Source: CAD feature listing. Evaluate the final solid. Frame: model axes, mm. Give positions to 0.01 mm unless a question says otherwise; leave off trailing zeros. Write each loop counter-clockwise with the first axis right and the second up, starting at its lowest first coordinate (ties: lowest second). Pieces come first, ordered by that corner, then holes. Notation, with made-up numbers: (42, 4.5) - (56, 4.5) arc R21 cw to (56, 25.5) - close; hole circle Ø2 at (-24.75, 70). An arc over 180 degrees is marked (long way). One line per question, with ' | ' between items. Start each with the question number.
(1) Section A-A, the plane x = -36.5. Return loops of the section in (y, z), plus the area to 3 significant figures.
(2) Ray query, line 1 (Z direction, x = -10.5, y = 1.5); line 2 (Z direction, x = 4, y = 1.85); line 3 (Z direction, x = 71, y = 0.5). Return the intervals inside material, ascending. Write a range as [from, to].
(3) Pin query (flat end, axial travel): pin 1 (4 mm diameter, centred on x = 14.5, z = 49.5, fed in from -Y). Return the tip coordinate at first contact, or that it passes through.
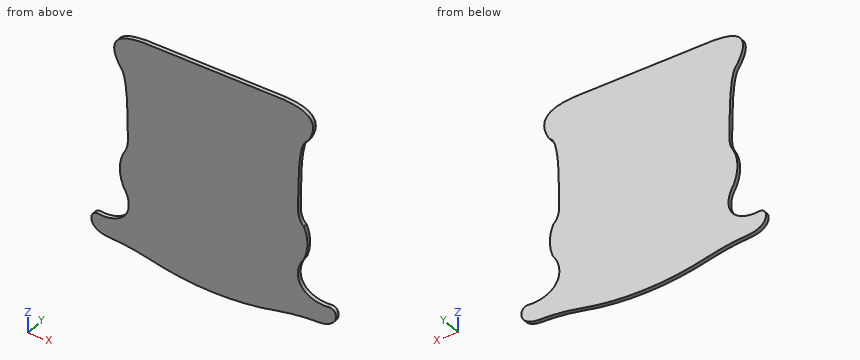
```python
from build123d import *

# Parameters (mm, degrees)
EXTRUDE_1_DEPTH = 3


with BuildPart() as part:
    # 草图1 → 凸台-拉伸1 (new body)
    with BuildSketch(Plane(origin=(0, 0, 0), x_dir=(1, 0, 0), z_dir=(0, 1, 0))):
        with BuildLine():
            Line((0, -85.237738925), (52.08455714, -85.237738925))
            add(Edge.make_bspline(
                [(52.08455714, -85.237738925), (83.131353316, -83.963442969), (70.531928888, -61.056271567)],
                knots=[0, 0, 0, 0.91576418, 0.91576418, 0.91576418], degree=2))
            add(Edge.make_bspline(
                [(64.686979765, -47.335345252), (64.821728452, -48.22885898), (65.093128633, -50.015668979), (65.515155467, -52.234660938), (65.946662506, -53.991070652), (66.337115564, -55.291267739), (66.823261096, -56.557684193), (67.433421369, -57.768689415), (68.186549634, -58.894674775), (69.089475072, -59.904951843), (69.899928779, -60.600614164), (70.397522986, -60.962598407), (70.531928888, -61.056271567)],
                knots=[0, 0, 0, 0, 0.03125, 0.0625, 0.078125, 0.09375, 0.109375, 0.125, 0.140625, 0.15625, 0.171875, 0.177544855, 0.177544855, 0.177544855, 0.177544855], degree=3))
            add(Edge.make_bspline(
                [(67.281190845, 5.878024568), (66.896150113, 5.604067681), (66.17820277, 4.954075775), (65.443341839, 3.984844748), (64.938700468, 3.142617887), (64.602832741, 2.486533462), (64.306406192, 1.811794699), (64.046527331, 1.122513569), (63.82116748, 0.421125393), (63.628358492, -0.290103239), (63.466128453, -1.008847892), (63.332437978, -1.733031566), (63.224920724, -2.461279505), (63.112896984, -3.436590381), (63.04248237, -4.416759867), (63.002674943, -5.39935773), (62.985358555, -6.136929173), (62.977857057, -6.874572053), (62.977765693, -7.612059791), (62.982878051, -8.349301424), (62.991452287, -9.086301707), (63.002218337, -9.823125162), (63.018489212, -10.805396372), (63.040788209, -12.033099303), (63.117509988, -15.961444796), (63.209965223, -19.888985412), (63.30476302, -23.816659201), (63.346660287, -25.535031616), (63.38326061, -27.007933212), (63.421035997, -28.480829039), (63.466381834, -30.199198036), (63.537017062, -32.653910516), (63.649386664, -35.598757346), (63.806392131, -38.54169042), (64.021636354, -41.480498428), (64.260256253, -43.924290625), (64.493829102, -45.874662228), (64.622628022, -46.848447014), (64.686979765, -47.335345252)],
                knots=[0.42243117, 0.42243117, 0.42243117, 0.42243117, 0.4375, 0.453125, 0.4609375, 0.46875, 0.4765625, 0.484375, 0.4921875, 0.5, 0.5078125, 0.515625, 0.5234375, 0.53125, 0.546875, 0.5546875, 0.5625, 0.5703125, 0.578125, 0.5859375, 0.59375, 0.6015625, 0.609375, 0.625, 0.640625, 0.734375, 0.75, 0.765625, 0.7890625, 0.796875, 0.8125, 0.84375, 0.875, 0.90625, 0.9375, 0.96875, 0.984375, 1, 1, 1, 1], degree=3))
            add(Edge.make_bspline(
                [(67.78565705, 30.270686681), (72.435451847, 17.336518953), (67.281190845, 5.878024568)],
                knots=[0.041125556, 0.041125556, 0.041125556, 0.901853171, 0.901853171, 0.901853171], degree=2))
            add(Edge.make_bspline(
                [(67.78565705, 30.270686681), (61.777966314, 38.050300603), (60.870236454, 48.571265725), (67.294682301, 54.787889309)],
                knots=[0.782114211, 0.782114211, 0.782114211, 0.782114211, 1, 1, 1, 1], degree=3))
            add(Edge.make_bspline(
                [(67.294682301, 54.787889309), (70.741983298, 58.123674712), (77.208516837, 60.562602986), (83.906576895, 60.259476119), (84.838000271, 60.163270829)],
                knots=[0, 0, 0, 0, 0.116915593, 0.136015961, 0.136015961, 0.136015961, 0.136015961], degree=3))
            add(Edge.make_bspline(
                [(84.838000271, 60.163270829), (85.146981152, 60.131356669), (85.454953169, 60.093539936), (85.761414982, 60.04983651)],
                knots=[0.136015961, 0.136015961, 0.136015961, 0.136015961, 0.142352122, 0.142352122, 0.142352122, 0.142352122], degree=3))
            add(Edge.make_bspline(
                [(78.685847617, 74.813097523), (82.796268879, 74.469500522), (85.960946813, 73.439665414), (92.408972751, 67.859232167), (92.136253049, 59.602987515), (85.761414982, 60.04983651)],
                knots=[0.020704184, 0.020704184, 0.020704184, 0.020704184, 0.398408746, 0.457074244, 0.967673839, 0.967673839, 0.967673839, 0.967673839], degree=3))
            ThreePointArc((78.685847617, 74.813097523), (62.72522618, 76.083545277), (46.990944234, 79.047975372))
            ThreePointArc((46.990944234, 79.047975372), (23.665112301, 83.299995302), (0, 84.761695887))
            Line((0, 84.761695887), (0, -85.237738925))
        make_face()
        with BuildLine():
            Line((-52.08455714, -85.237738925), (0, -85.237738925))
            Line((0, -85.237738925), (0, 84.761695887))
            ThreePointArc((0, 84.761695887), (-24.143998295, 83.356825814), (-47.941899914, 79.047975372))
            ThreePointArc((-47.941899914, 79.047975372), (-62.863562899, 76.194384461), (-77.997336876, 74.864763259))
            add(Edge.make_bspline(
                [(-77.997336876, 74.864763259), (-82.495528452, 74.563753901), (-85.819969627, 73.561673882), (-92.303254227, 67.950726086), (-92.148043047, 60.049699914), (-86.326016832, 60.03052313)],
                knots=[0, 0, 0, 0, 0.398408746, 0.457074244, 0.95214781, 0.95214781, 0.95214781, 0.95214781], degree=3))
            add(Edge.make_bspline(
                [(-84.476216485, 60.232119747), (-85.0964702, 60.188510883), (-85.714404489, 60.121269756), (-86.326016832, 60.03052313)],
                knots=[0.130603984, 0.130603984, 0.130603984, 0.130603984, 0.143267662, 0.143267662, 0.143267662, 0.143267662], degree=3))
            add(Edge.make_bspline(
                [(-67.726534157, 54.787889309), (-71.173835153, 58.123674712), (-77.383070006, 60.465559796), (-83.805773382, 60.279257331), (-84.476216485, 60.232119747)],
                knots=[0, 0, 0, 0, 0.116915593, 0.130603984, 0.130603984, 0.130603984, 0.130603984], degree=3))
            add(Edge.make_bspline(
                [(-67.318940817, 31.510044314), (-62.135044836, 39.136673255), (-61.6373547, 48.895686695), (-67.726534157, 54.787889309)],
                knots=[0.793484807, 0.793484807, 0.793484807, 0.793484807, 1, 1, 1, 1], degree=3))
            add(Edge.make_bspline(
                [(-67.318940817, 31.510044314), (-73.265342886, 16.40111188), (-65.978257792, 3.284039205)],
                knots=[0, 0, 0, 1, 1, 1], degree=2))
            add(Edge.make_bspline(
                [(-65.637935545, -47.335345136), (-65.373308793, -45.388720399), (-64.924382386, -41.484539572), (-64.643005293, -36.57962883), (-64.490248654, -32.653889947), (-64.374999228, -28.726358209), (-64.257498755, -23.816569768), (-64.116872777, -17.924883735), (-64.009829941, -13.015026184), (-63.947711012, -9.577682419), (-63.927494686, -7.612641533), (-63.933645618, -5.646217447), (-64.01771328, -3.681321264), (-64.270091341, -1.731417529), (-64.514844339, -0.526384591), (-64.771670226, 0.42231228), (-64.996859302, 1.123821794), (-65.256715294, 1.813004408), (-65.553427674, 2.487173233), (-65.802759649, 2.973687329), (-65.950639045, 3.235914899), (-65.978257792, 3.284039205)],
                knots=[0, 0, 0, 0, 0.0625, 0.125, 0.15625, 0.1875, 0.25, 0.3125, 0.375, 0.40625, 0.421875, 0.4375, 0.46875, 0.484375, 0.5, 0.5078125, 0.515625, 0.5234375, 0.53125, 0.5390625, 0.540827672, 0.540827672, 0.540827672, 0.540827672], degree=3))
            add(Edge.make_bspline(
                [(-67.844738769, -56.659038975), (-67.828076267, -56.622229396), (-67.719460833, -56.379300174), (-67.532147702, -55.924331546), (-67.301765295, -55.286577262), (-67.095120003, -54.640057247), (-66.846182809, -53.769830042), (-66.575335176, -52.672735761), (-66.298095135, -51.346567808), (-66.056394972, -50.013457449), (-65.839906621, -48.675631298), (-65.705201894, -47.782116323), (-65.637935545, -47.335345136)],
                knots=[0.889226319, 0.889226319, 0.889226319, 0.889226319, 0.890625, 0.8984375, 0.90625, 0.9140625, 0.921875, 0.9375, 0.953125, 0.96875, 0.984375, 1, 1, 1, 1], degree=3))
            add(Edge.make_bspline(
                [(-69.542046847, -59.335240196), (-69.41095783, -59.185836173), (-69.140909763, -58.858719517), (-68.761007501, -58.331544507), (-68.303961157, -57.600902177), (-68.014217124, -57.033438144), (-67.844738769, -56.659038975)],
                knots=[0.852481845, 0.852481845, 0.852481845, 0.852481845, 0.859375, 0.8671875, 0.875, 0.889226319, 0.889226319, 0.889226319, 0.889226319], degree=3))
            add(Edge.make_bspline(
                [(-52.08455714, -85.237738925), (-84.277652341, -83.916393856), (-69.542046847, -59.335240196)],
                knots=[0, 0, 0, 0.949575707, 0.949575707, 0.949575707], degree=2))
        make_face()
    extrude(amount=EXTRUDE_1_DEPTH)


solid = part.part
```
Check sheet entries:
1) outline: (0, -81.49) - (3, -81.49) - (3, 85.24) - (0, 85.24) - close | area: 500 mm²
2) line 1: [-84.51, 85.24] | line 2: [-84.71, 85.24] | line 3: [-75.21, -57.48], [61.93, 79.89]
3) pin 1: y = 0
